```python
from build123d import *

# Parameters (mm, degrees)
F0_W     = 152.5
F0_H     = 152.5
F0_R     = 2.55
F0_R_2   = 13.25
F1_DEPTH = 2


with BuildPart() as f1:
    # F0 (on Top) → F1 (new body)
    with BuildSketch(Plane.XY):
        Rectangle(F0_W, F0_H)
        with Locations((-72.2, -72.2)):
            Circle(F0_R, mode=Mode.SUBTRACT)
        with Locations((-60, -60)):
            Circle(F0_R_2, mode=Mode.SUBTRACT)
        with Locations((-30, -60)):
            Circle(F0_R_2, mode=Mode.SUBTRACT)
        with Locations((-60, -30)):
            Circle(F0_R_2, mode=Mode.SUBTRACT)
        with Locations((-45, -15)):
            Circle(F0_R, mode=Mode.SUBTRACT)
        with Locations((-30, -30)):
            Circle(F0_R_2, mode=Mode.SUBTRACT)
        with Locations((0, -60)):
            Circle(F0_R_2, mode=Mode.SUBTRACT)
        with Locations((30, -60)):
            Circle(F0_R_2, mode=Mode.SUBTRACT)
        with Locations((72.2, -72.2)):
            Circle(F0_R, mode=Mode.SUBTRACT)
        with Locations((60, -60)):
            Circle(F0_R_2, mode=Mode.SUBTRACT)
        with Locations((0, -30)):
            Circle(F0_R_2, mode=Mode.SUBTRACT)
        with Locations((30, -30)):
            Circle(F0_R_2, mode=Mode.SUBTRACT)
        with Locations((60, -30)):
            Circle(F0_R_2, mode=Mode.SUBTRACT)
        with Locations((45, -15)):
            Circle(F0_R, mode=Mode.SUBTRACT)
        with Locations((-60, 0)):
            Circle(F0_R_2, mode=Mode.SUBTRACT)
        with Locations((-45, 15)):
            Circle(F0_R, mode=Mode.SUBTRACT)
        with Locations((-60, 30)):
            Circle(F0_R_2, mode=Mode.SUBTRACT)
        with Locations((-30, 0)):
            Circle(F0_R_2, mode=Mode.SUBTRACT)
        with Locations((-30, 30)):
            Circle(F0_R_2, mode=Mode.SUBTRACT)
        with Locations((-60, 60)):
            Circle(F0_R_2, mode=Mode.SUBTRACT)
        with Locations((-72.2, 72.2)):
            Circle(F0_R, mode=Mode.SUBTRACT)
        with Locations((-30, 60)):
            Circle(F0_R_2, mode=Mode.SUBTRACT)
        Circle(F0_R_2, mode=Mode.SUBTRACT)
        with Locations((30, 0)):
            Circle(F0_R_2, mode=Mode.SUBTRACT)
        with Locations((0, 30)):
            Circle(F0_R_2, mode=Mode.SUBTRACT)
        with Locations((30, 30)):
            Circle(F0_R_2, mode=Mode.SUBTRACT)
        with Locations((45, 15)):
            Circle(F0_R, mode=Mode.SUBTRACT)
        with Locations((60, 0)):
            Circle(F0_R_2, mode=Mode.SUBTRACT)
        with Locations((60, 30)):
            Circle(F0_R_2, mode=Mode.SUBTRACT)
        with Locations((0, 60)):
            Circle(F0_R_2, mode=Mode.SUBTRACT)
        with Locations((30, 60)):
            Circle(F0_R_2, mode=Mode.SUBTRACT)
        with Locations((60, 60)):
            Circle(F0_R_2, mode=Mode.SUBTRACT)
        with Locations((72.2, 72.2)):
            Circle(F0_R, mode=Mode.SUBTRACT)
    extrude(amount=F1_DEPTH)


solid = f1.part
```
Geometry: final body of the model. Coordinates: model frame, mm. Round coordinates to 2 decimals unless told otherwise and drop trailing zeros. Order: outer loops, then holes, each group sorted by start corner. A loop starts at its lowest first (then second) coordinate and runs counter-clockwise, first axis right, second up. Notation, with made-up numbers: M 19.5,-39 L 60.5,-39 A15 ccw 60.5,-31 Z; hole C 83.5,-36 d4. An arc over 180 degrees is marked long. Use one line per item in the form item = value. Start each with the question number.
Q1. Cut plane C-C (z = 0.35). Count the separate pieces of the cut face and the enclosed holes in it, and give its area (3 significant figures).
Q2. Cut plane B-B (x = 19). Return loops of the section in (y, z).
Q3. Material intervals for line 1 (Y direction, x = 29, z = 1.8); line 2 (X direction, y = -0.5, z = 1.6); line 3 (Y direction, x = 45, z = 1.5), sorted ascending. Write a range as [from, to].
Q4. Cut plane A-A (y = 0). Return loops of the section in (x, z).
Geometry results:
q1.separate_pieces = 1
q1.enclosed_holes = 33
q1.area = 9,300 mm^2
q2.outline = M -76.25,0 L -67.39,0 L -67.39,2 L -76.25,2 Z; M -52.61,0 L -37.39,0 L -37.39,2 L -52.61,2 Z; M -22.61,0 L -7.39,0 L -7.39,2 L -22.61,2 Z; M 7.39,0 L 22.61,0 L 22.61,2 L 7.39,2 Z; M 37.39,0 L 52.61,0 L 52.61,2 L 37.39,2 Z; M 67.39,0 L 76.25,0 L 76.25,2 L 67.39,2 Z
q3.line_1 = [-76.25, -73.21], [-46.79, -43.21], [-16.79, -13.21], [13.21, 16.79], [43.21, 46.79], [73.21, 76.25]
q3.line_2 = [-76.25, -73.24], [-46.76, -43.24], [-16.76, -13.24], [13.24, 16.76], [43.24, 46.76], [73.24, 76.25]
q3.line_3 = [-76.25, -17.55], [-12.45, 12.45], [17.55, 76.25]
q4.outline = M -76.25,0 L -73.25,0 L -73.25,2 L -76.25,2 Z; M -46.75,0 L -43.25,0 L -43.25,2 L -46.75,2 Z; M -16.75,0 L -13.25,0 L -13.25,2 L -16.75,2 Z; M 13.25,0 L 16.75,0 L 16.75,2 L 13.25,2 Z; M 43.25,0 L 46.75,0 L 46.75,2 L 43.25,2 Z; M 73.25,0 L 76.25,0 L 76.25,2 L 73.25,2 Z
